from build123d import *

# Parameters (mm, degrees)
BOSS_EXTRUDE1_DEPTH     = 11
CUT_EXTRUDE2_DEPTH      = 8.05
BOSS_EXTRUDE2_REACH     = 38.858
SKETCH4_W               = 2.5
SKETCH4_H               = 1.5
BOSS_EXTRUDE5_DEPTH     = 3.05
FILLET3_R               = 1
SKETCH8_R               = 1.7
BOSS_EXTRUDE3_DEPTH     = 6
CHAMFER1_SIZE           = 2.5
CUT_EXTRUDE5_REACH      = 80.439
SKETCH10_R              = 1.7
BOSS_EXTRUDE4_DEPTH     = 9.6
CHAMFER3_SIZE           = 5
CHAMFER2_SIZE           = 1
CUT_EXTRUDE6_DEPTH      = 78.764773516
CUT_EXTRUDE6_DEPTH_BACK = 78.764773516
SKETCH15_R              = 1.5
CUT_EXTRUDE7_DEPTH      = 79.438526886


with BuildPart() as part:
    # Sketch1 → Boss-Extrude1 (new body)
    with BuildSketch(Plane.XY):
        with BuildLine():
            Line((1, 0), (19.7, 0))
            ThreePointArc((19.7, 0), (29.8, 10.1), (19.7, 20.2))
            Line((19.7, 20.2), (1, 20.2))
            ThreePointArc((1, 20.2), (0.292893219, 19.907106781), (0, 19.2))
            Line((0, 19.2), (0, 1))
            ThreePointArc((0, 1), (0.292893219, 0.292893219), (1, 0))
        make_face()
    extrude(amount=BOSS_EXTRUDE1_DEPTH)

    # Sketch3 → Cut-Extrude2 (cut)
    with BuildSketch(Plane.XY.offset(11)):
        with BuildLine():
            Line((0, 16), (19.7, 16))
            ThreePointArc((19.7, 16), (25.6, 10.1), (19.7, 4.2))
            Line((19.7, 4.2), (0, 4.2))
            Line((0, 4.2), (0, 16))
        make_face()
    extrude(amount=-CUT_EXTRUDE2_DEPTH, mode=Mode.SUBTRACT)

    # Sketch4 → Boss-Extrude2 (add, up to next)
    with BuildSketch(Plane.ZY.offset(-1), mode=Mode.PRIVATE) as boss_extrude2_sk1:
        with Locations((6.95, 15.25)):
            Rectangle(SKETCH4_W, SKETCH4_H)
    boss_extrude2_tool1 = extrude(boss_extrude2_sk1.sketch, amount=-BOSS_EXTRUDE2_REACH, mode=Mode.PRIVATE) - part.part
    # Sketch4 → Boss-Extrude2 (add, up to next)
    with BuildSketch(Plane.ZY.offset(-1), mode=Mode.PRIVATE) as boss_extrude2_sk2:
        with Locations((6.95, 4.95)):
            Rectangle(SKETCH4_W, SKETCH4_H)
    boss_extrude2_tool2 = extrude(boss_extrude2_sk2.sketch, amount=-BOSS_EXTRUDE2_REACH, mode=Mode.PRIVATE) - part.part
    add(boss_extrude2_tool1.solids().sort_by_distance((1, 15.25, 6.95))[0])
    add(boss_extrude2_tool2.solids().sort_by_distance((1, 4.95, 6.95))[0])

    # Sketch14 → Boss-Extrude5 (add)
    with BuildSketch(Plane.XY.offset(11)):
        with BuildLine():
            Line((0, 19.2), (0, 1))
            ThreePointArc((0, 1), (0.292893219, 0.292893219), (1, 0))
            Line((1, 0), (19.7, 0))
            ThreePointArc((19.7, 0), (29.8, 10.1), (19.7, 20.2))
            Line((19.7, 20.2), (1, 20.2))
            ThreePointArc((1, 20.2), (0.292893219, 19.907106781), (0, 19.2))
        make_face()
    extrude(amount=BOSS_EXTRUDE5_DEPTH)

    # Fillet3
    fillet3_edges = [part.edges().sort_by_distance(p)[0] for p in [
        (1, 15.25, 5.7),
        (1, 14.5, 6.95),
        (1, 15.25, 8.2),
        (1, 4.95, 5.7),
        (1, 4.95, 8.2),
        (1, 5.7, 6.95),
    ]]
    fillet(fillet3_edges, radius=FILLET3_R)

    # Sketch8 → Boss-Extrude3 (add)
    with BuildSketch(Plane(origin=(0, 0, 14.05), x_dir=(-1, 0, 0), z_dir=(0, 0, -1))):
        with BuildLine():
            Line((-19.7, 25.6), (-72.8, 25.6))
            Line((-72.8, 25.6), (-72.8, -5.4))
            Line((-72.8, -5.4), (-19.7, -5.4))
            Line((-19.7, -5.4), (-19.7, 4.2))
            ThreePointArc((-19.7, 4.2), (-25.6, 10.1), (-19.7, 16))
            Line((-19.7, 16), (-19.7, 25.6))
        make_face()
        with Locations((-64.8, 10.1)):
            Circle(SKETCH8_R, mode=Mode.SUBTRACT)
        with Locations((-56.8, 2.1)):
            Circle(SKETCH8_R, mode=Mode.SUBTRACT)
        with Locations((-48.8, 10.1)):
            Circle(SKETCH8_R, mode=Mode.SUBTRACT)
        with Locations((-56.8, 18.1)):
            Circle(SKETCH8_R, mode=Mode.SUBTRACT)
    extrude(amount=BOSS_EXTRUDE3_DEPTH)

    # Chamfer1
    chamfer1_edges = [part.edges().sort_by_distance(p)[0] for p in [
        (19.7, -5.4, 11.05),
        (19.7, 25.6, 11.05),
        (72.8, 25.6, 11.05),
        (72.8, -5.4, 11.05),
    ]]
    chamfer(chamfer1_edges, length=CHAMFER1_SIZE)

    # Sketch10 → Cut-Extrude5 (cut, up to next)
    with BuildSketch(Plane(origin=(0, 0, 0), x_dir=(-1, 0, 0), z_dir=(0, 0, -1)), mode=Mode.PRIVATE) as cut_extrude5_sk1:
        with Locations((-7.5, 10.1)):
            Circle(SKETCH10_R)
    cut_extrude5_tool1 = extrude(cut_extrude5_sk1.sketch, amount=-CUT_EXTRUDE5_REACH, mode=Mode.PRIVATE) & part.part
    # Sketch10 → Cut-Extrude5 (cut, up to next)
    with BuildSketch(Plane(origin=(0, 0, 0), x_dir=(-1, 0, 0), z_dir=(0, 0, -1)), mode=Mode.PRIVATE) as cut_extrude5_sk2:
        with Locations((-19.5, 10.1)):
            Circle(SKETCH10_R)
    cut_extrude5_tool2 = extrude(cut_extrude5_sk2.sketch, amount=-CUT_EXTRUDE5_REACH, mode=Mode.PRIVATE) & part.part
    add(cut_extrude5_tool1.solids().sort_by_distance((7.5, 10.1, 0))[0], mode=Mode.SUBTRACT)
    add(cut_extrude5_tool2.solids().sort_by_distance((19.5, 10.1, 0))[0], mode=Mode.SUBTRACT)

    # Sketch11 → Boss-Extrude4 (add)
    with BuildSketch(Plane(origin=(0, 0, 8.05), x_dir=(-1, 0, 0), z_dir=(0, 0, -1))):
        Polygon((-22.2, 25.6), (-70.3, 25.6), (-72.8, 23.1), (-72.8, -2.9), (-70.3, -5.4), (-22.2, -5.4), (-22.2, -2.4), (-68.8, -2.4), (-69.8, -1.4), (-69.8, 21.6), (-68.8, 22.6), (-22.2, 22.6), align=None)
    extrude(amount=BOSS_EXTRUDE4_DEPTH)

    # Chamfer3
    chamfer3_edges = [part.edges().sort_by_distance(p)[0] for p in [
        (22.2, 24.1, -1.55),
        (22.2, -3.9, -1.55),
    ]]
    chamfer(chamfer3_edges, length=CHAMFER3_SIZE)

    # Chamfer2
    chamfer2_edges = [part.edges().sort_by_distance(p)[0] for p in [
        (48.75, 25.6, -1.55),
        (46.25, -5.4, 14.05),
        (72.8, 10.1, 14.05),
        (72.8, 10.1, -1.55),
        (46.25, 25.6, 14.05),
        (22.2, 25.6, 5.75),
        (22.2, -5.4, 5.75),
        (24.7, -5.4, 0.95),
        (24.7, 25.6, 0.95),
        (48.75, -5.4, -1.55),
        (71.55, -4.15, -1.55),
        (71.55, 24.35, -1.55),
        (10.35, 0, 0),
        (29.8, 10.1, 0),
        (10.35, 20.2, 0),
        (0.292893219, 19.907106781, 0),
        (0.292893219, 0.292893219, 0),
        (0, 10.1, 0),
        (0, 10.1, 14.05),
        (10.35, 0, 14.05),
        (19.7, -1.45, 14.05),
        (20.95, -4.15, 14.05),
        (0.292893219, 0.292893219, 14.05),
        (0.292893219, 19.907106781, 14.05),
        (10.35, 20.2, 14.05),
        (19.7, 21.65, 14.05),
        (20.95, 24.35, 14.05),
    ]]
    chamfer(chamfer2_edges, length=CHAMFER2_SIZE - 0.0001)  # a hair under: the kernel refuses the full size

    # Sketch12 → Cut-Extrude6 (cut, two sides: drawn at the far end of the back side and taken through both)
    with BuildSketch(Plane(origin=(0, 0, 8.05), x_dir=(-1, 0, 0), z_dir=(0, 0, -1)).offset(-CUT_EXTRUDE6_DEPTH_BACK)):
        Polygon((-38.2, 4.6), (-38.2, 15.6), (-36.2, 17.6), (-32.2, 17.6), (-30.2, 15.6), (-30.2, 4.6), (-32.2, 2.6), (-36.2, 2.6), align=None)
    extrude(amount=CUT_EXTRUDE6_DEPTH + CUT_EXTRUDE6_DEPTH_BACK, mode=Mode.SUBTRACT)

    # Sketch15 → Cut-Extrude7 (cut, through all)
    with BuildSketch(Plane(origin=(0, 0, 0), x_dir=(-1, 0, 0), z_dir=(0, 0, -1))):
        with Locations((-19.5, 10.1)):
            Circle(SKETCH15_R)
        with Locations((-7.5, 10.1)):
            Circle(SKETCH15_R)
    extrude(amount=-CUT_EXTRUDE7_DEPTH, mode=Mode.SUBTRACT)


solid = part.part
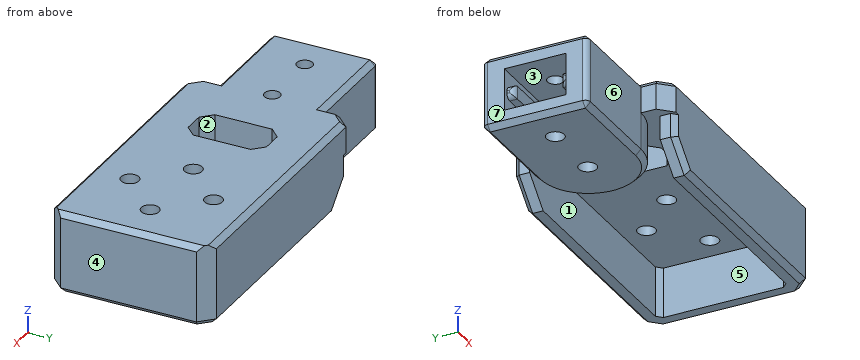
Model file for the job. Use its own axes, mm. Face numbers are marked on the shaded views. A direction names the side the tool comes from. Give positions to 0.01 mm unless a question says otherwise; leave off trailing zeros. Order: outer loops, then holes, each group sorted by start corner. A loop starts at its lowest first (then second) coordinate and runs counter-clockwise, first axis right, second up. Notation, with made-up numbers: (32, 69) -> (59, 69) arc R22 cw to (59, 75) -> close; hole circle Ø11 at (61.25, 12). An arc over 180 degrees is marked (long way). Use CSV: the item, a comma, the result in double quotes.
1. 3-axis set-ups, long thin cutter, end or side, ignore diameter. For the marked faces 1, 2 and 3: which of +Z, -Z, +X, -X, +Y, -Y reach the whole face in a straight line?
Outcome:
face 1,"-Z, -X"
face 2,"+Z, -Z"
face 3,"-X"
2. Drop flat-ended pins along their axis: pin 1 (6 mm diameter, centred on x = 8.5, z = 8, fed in from -Y); pin 2 (10 mm diameter, centred on x = 35.5, y = 17.5, fed in from -Z); pin 3 (4.5 mm diameter, centred on x = 64.8, y = 10.1, fed in from -Z); pin 4 (2 mm diameter, centred on x = 19.5, y = 10.1, fed in from -Z) (3 decimals). Give the stop position or say it passes through.
Outcome:
pin 1,"y = 0"
pin 2,"z = 8.05"
pin 3,"z = 8.05"
pin 4,"through"
3. Band-saw the part on C-C, the plane z = 9. Count the separate pieces of the cut face and the enclosed holes in it, then the cut area to 3 significant figures.
Outcome:
separate pieces,"1"
enclosed holes,"5"
area,"1,600 mm²"
4. Band-saw the part on B-B, the plane x = 7.5. Give the cut face in (y, z), then the cut area to 3 significant figures.
Outcome:
outline,"(0, 1) -> (1, 0) -> (8.4, 0) -> (8.4, 2.95) -> (4.2, 2.95) -> (4.2, 5.7) -> (5.7, 5.7) -> (5.7, 8.2) -> (4.2, 8.2) -> (4.2, 11) -> (8.6, 11) -> (8.6, 14.05) -> (1, 14.05) -> (0, 13.05) -> close; (11.6, 11) -> (16, 11) -> (16, 8.2) -> (14.5, 8.2) -> (14.5, 5.7) -> (16, 5.7) -> (16, 2.95) -> (11.8, 2.95) -> (11.8, 0) -> (19.2, 0) -> (20.2, 1) -> (20.2, 13.05) -> (19.2, 14.05) -> (11.6, 14.05) -> close"
area,"175 mm²"
5. Band-saw the part on A-A, the plane z = 12. Give the cut face in (x, y).
Outcome:
outline,"(0, 1) arc R1 ccw to (1, 0) -> (19.7, 0) -> (19.7, -2.9) -> (22.2, -5.4) -> (70.3, -5.4) -> (72.8, -2.9) -> (72.8, 23.1) -> (70.3, 25.6) -> (22.2, 25.6) -> (19.7, 23.1) -> (19.7, 20.2) -> (1, 20.2) arc R1 ccw to (0, 19.2) -> close; hole circle Ø3 at (7.5, 10.1); hole circle Ø3 at (19.5, 10.1); hole (30.2, 4.6) -> (32.2, 2.6) -> (36.2, 2.6) -> (38.2, 4.6) -> (38.2, 15.6) -> (36.2, 17.6) -> (32.2, 17.6) -> (30.2, 15.6) -> close; hole circle Ø3.4 at (48.8, 10.1); hole circle Ø3.4 at (56.8, 2.1); hole circle Ø3.4 at (56.8, 18.1); hole circle Ø3.4 at (64.8, 10.1)"
6. Drill centre lines: line 1 along Y through (x, z) = (56.8, 10.6); line 2 along Y through (x, z) = (32.5, 8.75); line 3 along Y through (x, z) = (64.8, 12). Where is each one in solid material? Low to high. Write a range as from..to.
Outcome:
line 1,"-5.4..0.4, 3.8..16.4, 19.8..25.6"
line 2,"-5.4..2.6, 17.6..25.6"
line 3,"-5.4..8.4, 11.8..25.6"
7. Mould opens along X. For the marked faces 4, 5, 6 and 7 say: +X half, -X half, draft (parallel to the pull), parting line (faces both ways), or undercut.
Outcome:
face 4,"+X half"
face 5,"undercut"
face 6,"draft"
face 7,"-X half"
